Source: three-view drawing plus pictorial views. Frame: mm from the lowest corner of the part. A direction names the side the tool comes from. Coordinates: 2 decimals unless noted, no trailing zeros. Write each loop counter-clockwise with the first axis right and the second up, starting at its lowest first coordinate (ties: lowest second). Pieces come first, ordered by that corner, then holes. Notation, with made-up numbers: (5.5, 61) - (14.5, 61) arc R18 ccw to (14.5, 95) - close; hole circle Ø3 at (85.25, 30). An arc over 180 degrees is marked (long way). Put each result on its own line as item: value.
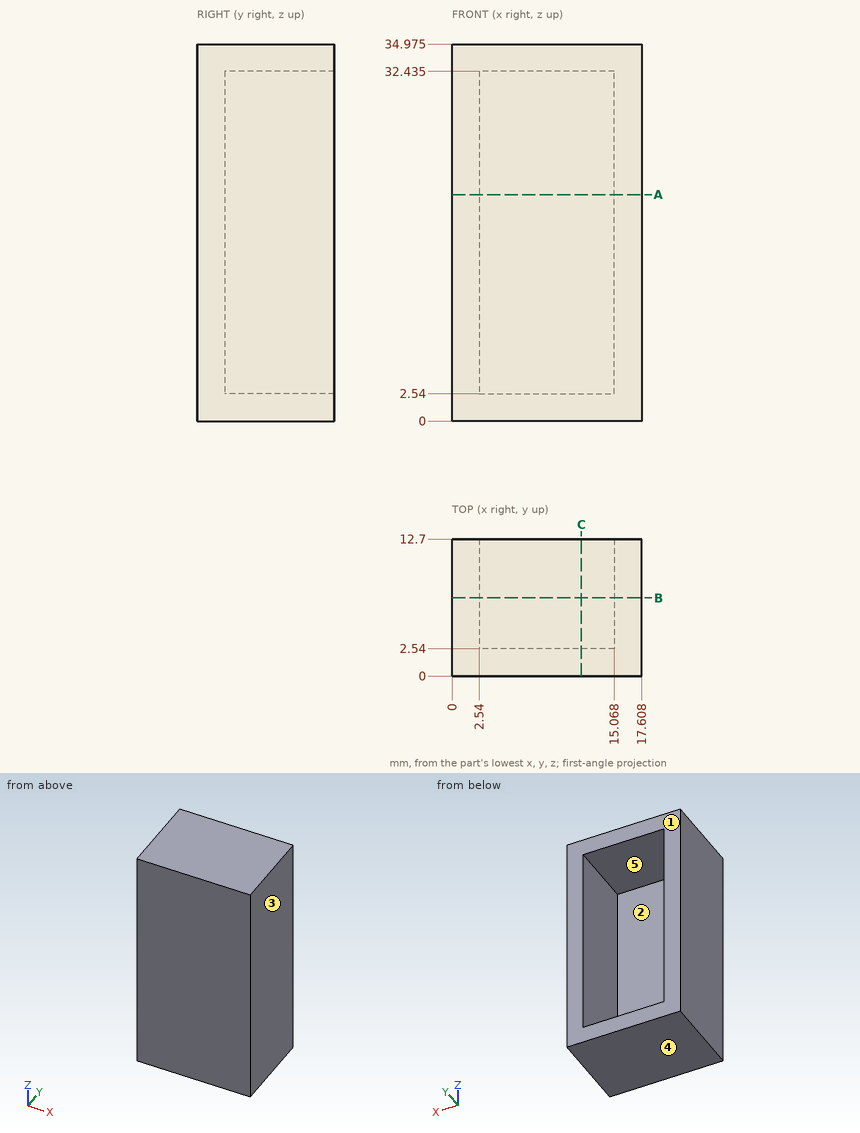
1. Section query A-A (z = 21). Return loops of the section in (x, y).
Answer below:
outline: (0, 0) - (17.61, 0) - (17.61, 12.7) - (15.07, 12.7) - (15.07, 2.54) - (2.54, 2.54) - (2.54, 12.7) - (0, 12.7) - close
2. Ray query, probe 1 along X at (y, z) = (6.25, 24.5); probe 2 along Z at (x, y) = (11.75, 10.75) (1 decimal); probe 3 along Y at (x, z) = (5, 20.5). Return the intervals inside material, ascending. Write a range as from..to.
Answer below:
probe 1: x = 0..2.54, 15.07..17.61
probe 2: z = 0..2.5, 32.4..35
probe 3: y = 0..2.54
3. Set-up query: the marked faces 4 and 5. Return all of +Z, -Z, +X, -X, +Y, -Y with unobstructed straight access to the full face (end or side cutting, diameter ignored); none if empty.
Answer below:
face 4: -Z, +X, -X, +Y, -Y
face 5: +Y
4. Pin query (flat end, axial travel): pin 1 Ø8 at (x, z) = (5.5, 27) entering from +Y; pin 2 Ø3 at (x, z) = (13, 30.5) entering from +Y. Return the tip coordinate at first contact, or that it passes through.
Answer below:
pin 1: stops at y = 12.7
pin 2: stops at y = 2.54
5. Section query B-B (y = 7.25). Return loops of the section in (x, z) (1 decimal).
Answer below:
outline: (0, 0) - (17.6, 0) - (17.6, 35) - (0, 35) - close; hole (2.5, 2.5) - (15.1, 2.5) - (15.1, 32.4) - (2.5, 32.4) - close
6. Mould query, pull axis X, two halves, no side actions, for the marked faces 1, 2 and 3. Classes: +X half, -X half, draft (parallel to the pull), parting line (faces both ways), or undercut.
Answer below:
face 1: draft
face 2: undercut
face 3: +X half
7. Section query C-C (x = 12). Return loops of the section in (y, z) (1 decimal).
Answer below:
outline: (0, 0) - (12.7, 0) - (12.7, 2.5) - (2.5, 2.5) - (2.5, 32.4) - (12.7, 32.4) - (12.7, 35) - (0, 35) - close
